from build123d import *

# Parameters (mm, degrees)
ESQUISSE1_R      = 13
EXTRUSION1_DEPTH = 0.5
ESQUISSE2_R      = 10.875
EXTRUSION2_DEPTH = 9
ESQUISSE3_R      = 13
EXTRUSION3_DEPTH = 0.5
ESQUISSE4_R      = 8
EXTRUSION4_DEPTH = 6
ESQUISSE5_R      = 2.5
EXTRUSION5_DEPTH = 25.372115214


with BuildPart() as part:
    # Esquisse1 → Extrusion1 (new body)
    with BuildSketch(Plane.XY):
        Circle(ESQUISSE1_R)
    extrude(amount=EXTRUSION1_DEPTH)

    # Esquisse2 → Extrusion2 (add)
    with BuildSketch(Plane.XY.offset(0.5)):
        Circle(ESQUISSE2_R)
    extrude(amount=EXTRUSION2_DEPTH)

    # Esquisse3 → Extrusion3 (add)
    with BuildSketch(Plane.XY.offset(9.5)):
        Circle(ESQUISSE3_R)
    extrude(amount=EXTRUSION3_DEPTH)

    # Esquisse4 → Extrusion4 (add)
    with BuildSketch(Plane.XY.offset(10)):
        Circle(ESQUISSE4_R)
    extrude(amount=EXTRUSION4_DEPTH)

    # Esquisse5 → Extrusion5 (cut, through all)
    with BuildSketch(Plane.XY.offset(16)):
        Circle(ESQUISSE5_R)
    extrude(amount=-EXTRUSION5_DEPTH, mode=Mode.SUBTRACT)


solid = part.part
Can you work these out from the model? Positions are in its coordinate system, mm. A direction names the side the tool comes from. Give positions to 0.01 mm unless a question says otherwise; leave off trailing zeros. Order: outer loops, then holes, each group sorted by start corner. A loop starts at its lowest first (then second) coordinate and runs counter-clockwise, first axis right, second up. Notation, with made-up numbers: M 20,53 L 66,53 A7 ccw 66,59 Z; hole C 52,-10.75 d5. An arc over 180 degrees is marked long. Use a Markdown table: item, result. Add a question column.
Item 1: Suppose I cut it at D-D (y = 10.25). List the corners of the cut face in (x, z) for me.
Item 2: Suppose I cut it at A-A (y = 0). List the corners of the cut face in (x, z) for me (3 decimals), then the cut area to 3 significant figures.
Item 3: We'd pull the mould along X, two halves only. Please class faces 1 (the cylindrical face through (-0.54, -2.44, 8.11)), 2 (the cylindrical face through (-1.73, -7.81, 12.96)), 3 (the flat face through (3, 0, 0)): +X half, -X half, draft (parallel to the pull), parting line (faces both ways), or undercut.
Item 4: Will these pins go through, and if not, where does the flat tip stop? pin 1 (3 mm diameter, centred on x = 2.5, z = 9, fed in from +Y); pin 2 (6 mm diameter, centred on x = -10, z = 5, fed in from +Y); pin 3 (2 mm diameter, centred on x = 7.5, z = 3, fed in from -Y).
Item 5: Suppose I cut it at C-C (z = 10.5). List the corners of the cut face in (x, y) for me, then the cut area to 3 significant figures.
Item 6: If I drill on L1, parallel to Z at x = -9.5, y = -5.5; L2, parallel to Y at x = 0, z = 6.25 (3 decimals); L3, parallel to Z at x = -9, y = 1, over which ranges is the centre line in solid material (lowest first)? Write a range as [from, to].
Item 7: For faces 4 (the flat face through (-3, -11, 9.5)), 5 (the cylindrical face through (-10.316, -7.91, 9.746)), 6 (the flat face through (6, 6, 10)), which set-ups out of +Z, -Z, +X, -X, +Y, -Y let a thin tool reach every point of the face, with its end or its side?
Answer sheet:
| question | item | result |
|---|---|---|
| 1 | outline | M -8,0 L 8,0 L 8,0.5 L 3.63,0.5 L 3.63,9.5 L 8,9.5 L 8,10 L -8,10 L -8,9.5 L -3.63,9.5 L -3.63,0.5 L -8,0.5 Z |
| 2 | outline | M -13,0 L -2.5,0 L -2.5,16 L -8,16 L -8,10 L -13,10 L -13,9.5 L -10.875,9.5 L -10.875,0.5 L -13,0.5 Z; M 2.5,0 L 13,0 L 13,0.5 L 10.875,0.5 L 10.875,9.5 L 13,9.5 L 13,10 L 8,10 L 8,16 L 2.5,16 Z |
| 2 | area | 238 mm² |
| 3 | face 1 | undercut |
| 3 | face 2 | parting line |
| 3 | face 3 | draft |
| 4 | pin 1 | stops at y = 12.95 |
| 4 | pin 2 | stops at y = 8.32 |
| 4 | pin 3 | stops at y = -8.72 |
| 5 | outline | C 0,0 d16; hole C 0,0 d5 |
| 5 | area | 181 mm² |
| 6 | L1 | z = [0, 0.5], [9.5, 10] |
| 6 | L2 | y = [-10.875, -2.5], [2.5, 10.875] |
| 6 | L3 | z = [0, 10] |
| 7 | face 4 | none |
| 7 | face 5 | +Z, -Z |
| 7 | face 6 | +Z |
